```python
from build123d import *

# Parameters (mm, degrees)
SKETCH1_R           = 10
BOSS_EXTRUDE1_DEPTH = 3
FILLET1_R           = 5


with BuildPart() as part:
    # Sketch1 → Boss-Extrude1 (new body)
    with BuildSketch(Plane(origin=(0, 0, 0), x_dir=(1, 0, 0), z_dir=(0, 1, 0))):
        Polygon((10, -20), (30, -20), (30, 20), (-30, 20), (-30, -20), (-10, -20), (-10, -17), (10, -17), align=None)
        with Locations(Location((-10.5, 0, 0), (0, 0, 270))):
            Circle(SKETCH1_R, mode=Mode.SUBTRACT)
    extrude(amount=BOSS_EXTRUDE1_DEPTH)

    # Fillet1
    fillet1_edges = [part.edges().sort_by_distance(p)[0] for p in [
        (-30, 1.5, -20),
        (30, 1.5, -20),
    ]]
    fillet(fillet1_edges, radius=FILLET1_R)


solid = part.part
```
Design review of the part built by this model. Coordinates are the model's own, in mm. A direction names the side the tool comes from. Coordinates: 2 decimals unless noted, no trailing zeros. Order: outer loops, then holes, each group sorted by start corner. A loop starts at its lowest first (then second) coordinate and runs counter-clockwise, first axis right, second up.
1) Wall thickness on line 1 along X through (y, z) = (2.45, 0); line 2 along X through (y, z) = (2.8, 18); line 3 along Z through (x, y) = (5, 1.6): over which ranges is each line inside the solid? List them lowest first.
2) Clearance check with a flat-ended pin moving along its axis: pin 1 (12 mm diameter, centred on x = 18.5, z = 14.5, fed in from -Y). State where the tip first meets the part, or that it passes through.
3) Take a section at B-B, the plane y = 2.25. Give the boundary of the cut face in (x, z).
4) Mouldability with a two-part tool opening along X and no side actions: class faces 3 (the flat face through (0, 1, 17)), 4 (the flat face through (30, 1, 3)), 5 (the flat face through (-20, 1, 20)), 6 (the flat face through (-10, 1, 19)) as +X half, -X half, draft (parallel to the pull), parting line (faces both ways), or undercut.
5) Take a section at C-C, the plane x = -17. Give the boundary of the cut face in (y, z), and give its area (3 significant figures).
6) For faces 1 (the flat face through (10, 1, 18)), 2 (the flat face through (20, 1, 20)), list the 3-axis set-ups (+Z, -Z, +X, -X, +Y, -Y) from which the entire face can be reached by the end or side of a thin tool; tool diameter is ignored.
7) Take a section at A-A, the plane z = 0. Give the boundary of the cut face in (x, y).
Returned:
1. line 1: x = -30 to -20.5, -0.5 to 30
1. line 2: x = -30 to -10, 10 to 30
1. line 3: z = -20 to 17
2. pin 1: stops at y = 0
3. outline: (-30, -15) arc R5 ccw to (-25, -20) - (25, -20) arc R5 ccw to (30, -15) - (30, 20) - (10, 20) - (10, 17) - (-10, 17) - (-10, 20) - (-30, 20) - close; hole circle Ø20 at (-10.5, 0)
4. face 3: undercut
4. face 4: +X half
4. face 5: draft
4. face 6: undercut
5. outline: (0, -20) - (3, -20) - (3, -7.6) - (0, -7.6) - close; (0, 7.6) - (3, 7.6) - (3, 20) - (0, 20) - close
5. area: 74.4 mm2
6. face 1: +Z, +Y, -Y
6. face 2: +Z, +X, -X, +Y, -Y
7. outline: (-30, 0) - (-20.5, 0) - (-20.5, 3) - (-30, 3) - close; (-0.5, 0) - (30, 0) - (30, 3) - (-0.5, 3) - close
